CAD build for the part. Positions are in the model's coordinates, mm. Coordinates: 2 decimals unless noted, no trailing zeros. Order: outer loops, then holes, each group sorted by start corner. A loop starts at its lowest first (then second) coordinate and runs counter-clockwise, first axis right, second up. Notation, with made-up numbers: (44.5, -8) - (99.5, -8) arc R13 ccw to (99.5, 14) - close; hole circle Ø11 at (28.5, 58). An arc over 180 degrees is marked (long way). Write each question's results on one line, items separated by ' | '. Start each with the question number.
Q1. Band-saw the part on C-C, the plane z = -129.5. Write the cut outline in (x, y).
Q2. Band-saw the part on A-A, the plane y = 1.15. Write the cut outline in (x, z).
Q3. Band-saw the part on B-B, the plane x = -48.5. Write the cut outline in (y, z).
Q4. Wall check: probe 1 along Z at (x, y) = (-27, 0.6); probe 2 along X at (y, z) = (0.2, -208). Give the ranges that are in metal, low to high.
Q5. Pin check, flat tips, straight feed: P1, Ø0.6, axis at x = -59.5, y = 0.5, coming from the -Z side; P2, Ø1, axis at y = 1, z = -41, coming from the -X side. Stop position of each tip, or through.
Autodesk Inventor part; units mm, degrees
ref_plane "YZ Plane" through (0, 0, 0) normal (1, 0, 0) x (0, 1, 0)
ref_plane "XZ Plane" through (0, 0, 0) normal (0, 1, 0) x (-1, 0, 0)
ref_plane "XY Plane" through (0, 0, 0) normal (0, 0, 1) x (1, 0, 0)
sketch "Sketch1" plane through (0, 0, 0) normal (0, 1, 0) x (-1, 0, 0)
  line L0 (5, -525) -> (-90, -525)
  line L1 (-90, 525) -> (90, 525)
  line L2 (0, 525) -> (0, -525)
  line L3 (5, -525) -> (5, 125)
  line L4 (5, 125) -> (90, 125)
  line L5 (90, 525) -> (90, 125)
  line L6 (5, 0) -> (-90, 0)
  line L7 (-90, 525) -> (-90, -525)
  point P0 (0, 0)
  dimension "d6" = 1050
  dimension "d7" = 180
  dimension "d8" = 85
  dimension "d10" = 650
extrude "Extrusion1" add sketch "Sketch1" along normal blind 2
properties part number "Si" material "LCP Plastic"
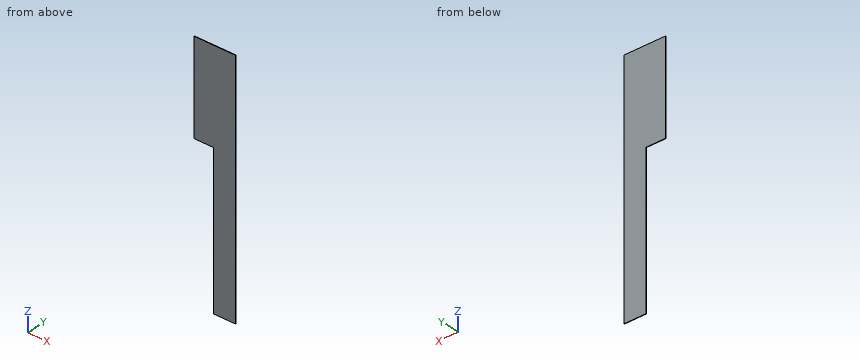
Results below:
1) outline: (-5, 0) - (90, 0) - (90, 2) - (-5, 2) - close
2) outline: (-90, 125) - (-5, 125) - (-5, -525) - (90, -525) - (90, 525) - (-90, 525) - close
3) outline: (0, 125) - (2, 125) - (2, 525) - (0, 525) - close
4) probe 1: z = 125 to 525 | probe 2: x = -5 to 90
5) P1: stops at z = 125 | P2: stops at x = -5
